from build123d import *

# Parameters (mm, degrees)
F1_DEPTH = 36
F3_DEPTH = 20.001


with BuildPart() as f1:
    # F0 (on Top) → F1 (new body)
    with BuildSketch(Plane.XY):
        Polygon((0, 20), (0, 0), (10, 0), (10, 8), (28, 8), (28, 20), align=None)
    extrude(amount=F1_DEPTH)

    # F2 (on Front) → F3 (cut, through all)
    with BuildSketch(Plane.XZ):
        Polygon((24.248711, 36), (0, 36), (0, 22), align=None)
    extrude(amount=-F3_DEPTH, mode=Mode.SUBTRACT)


solid = f1.part
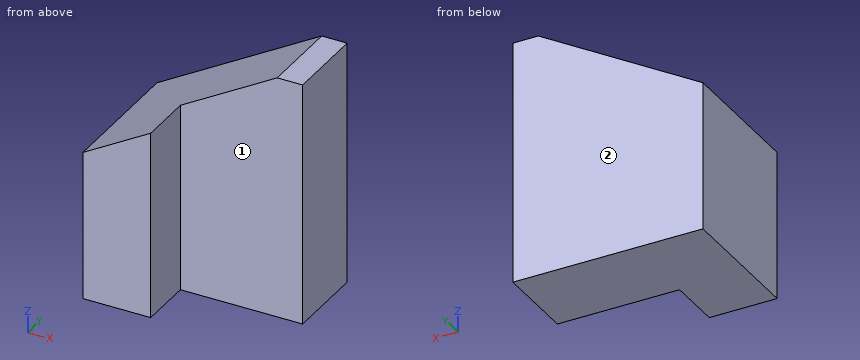
Work out the finished part from the listing and answer in its coordinate system (mm). Face numbers are marked on the shaded views. A direction names the side the tool comes from. Coordinates: 2 decimals unless noted, no trailing zeros. Write each loop counter-clockwise with the first axis right and the second up, starting at its lowest first coordinate (ties: lowest second). Pieces come first, ordered by that corner, then holes. Notation, with made-up numbers: M -29.75,73.5 L 17.25,73.5 A18 cw 17.25,102.5 Z; hole C 17.25,81.25 d5. An arc over 180 degrees is marked long. Write item = value, one per line.
1. The part is cut by section C-C (x = 7.75). Determine the outline of the cut face in (y, z).
Solution:
outline = M 0,0 L 20,0 L 20,26.47 L 0,26.47 Z
2. For the marked faces 1 and 2, determine the directions among +Z, -Z, +X, -X, +Y, -Y from which every point of the face is accessible in a straight line to the end or side of a thin tool.
Solution:
face_1 = +Z, -Z, +X, -Y
face_2 = +Z, -Z, +X, -X, +Y
3. The part is cut by section A-A (y = 4). Determine the outline of the cut face in (x, z), then the cut area to 3 significant figures.
Solution:
outline = M 0,0 L 10,0 L 10,27.77 L 0,22 Z
area = 249 mm2
4. Straight lines are drawn through the part: line 1 (X direction, y = 2, z = 9.5); line 2 (Y direction, x = 11.5, z = 6); line 3 (Z direction, x = 17, y = 11.5). For each, find the intervals that lie inside material, in ascending order. Write a range as from..to.
Solution:
line_1 = 0..10
line_2 = 8..20
line_3 = 0..31.81
5. The part is cut by section B-B (z = 13.5). Determine the outline of the cut face in (x, y).
Solution:
outline = M 0,0 L 10,0 L 10,8 L 28,8 L 28,20 L 0,20 Z
6. Flat-ended cylindrical pins translate along their axes: pin 1 (3 mm diameter, centred on x = 23.5, z = 30, fed in from -Y); pin 2 (1 mm diameter, centred on x = 3.5, y = 5.5, fed in from +Z); pin 3 (1.5 mm diameter, centred on x = 8.5, y = 7.5, fed in from +Z). Find the tip coordinate at first contact, or state that the pin passes through.
Solution:
pin_1 = 8
pin_2 = 24.31
pin_3 = 27.34
7. The part is cut by section D-D (y = 16.5). Determine the outline of the cut face in (x, z).
Solution:
outline = M 0,0 L 28,0 L 28,36 L 24.25,36 L 0,22 Z
